```python
from build123d import *

# Parameters (mm, degrees)
F0_W     = 490
F0_H     = 6
F1_DEPTH = 50


# Not quite as in the source:
# - a feature names something its author has since deleted; it is built from what else it names
# - the program builds the solid bodies; features that only make, move or delete a surface that nothing else refers to are left out


with BuildPart() as f1:
    # F0 (on Top) → F1 (new body)
    with BuildSketch(Plane.XY):
        Polygon((0, 1190), (0, 0), (515, 0), (540, 0), (540, 25), (540, 125), (540, 131), (540, 539), (540, 545), (540, 645), (540, 651), (540, 1059), (540, 1065), (540, 1165), (540, 1190), (515, 1190), align=None)
        Polygon((25, 1065), (25, 1165), (515, 1165), (515, 1065), (515, 1059), (515, 651), (515, 645), (515, 545), (515, 539), (515, 131), (515, 125), (515, 25), (25, 25), (25, 125), (25, 131), (25, 539), (25, 545), (25, 645), (25, 651), (25, 1059), align=None, mode=Mode.SUBTRACT)
        Polygon((540, 25), (540, 0), (1030, 0), (1055, 0), (1055, 25), (1055, 125), (1055, 131), (1055, 539), (1055, 545), (1055, 645), (1055, 651), (1055, 1059), (1055, 1065), (1055, 1165), (1055, 1190), (1030, 1190), (540, 1190), (540, 1165), (1030, 1165), (1030, 1065), (1030, 1059), (1030, 651), (1030, 645), (1030, 545), (1030, 539), (1030, 131), (1030, 125), (1030, 25), align=None)
        Polygon((1055, 25), (1055, 0), (1545, 0), (1570, 0), (1570, 25), (1570, 125), (1570, 131), (1570, 539), (1570, 545), (1570, 645), (1570, 651), (1570, 1059), (1570, 1065), (1570, 1165), (1570, 1190), (1545, 1190), (1055, 1190), (1055, 1165), (1545, 1165), (1545, 1065), (1545, 1059), (1545, 651), (1545, 645), (1545, 545), (1545, 539), (1545, 131), (1545, 125), (1545, 25), align=None)
        Polygon((1570, 25), (1570, 0), (2085, 0), (2085, 1190), (1570, 1190), (1570, 1165), (2060, 1165), (2060, 1065), (2060, 1059), (2060, 651), (2060, 645), (2060, 545), (2060, 539), (2060, 131), (2060, 125), (2060, 25), align=None)
        with Locations((270, 542)):
            Rectangle(F0_W, F0_H)
        with Locations((270, 128)):
            Rectangle(F0_W, F0_H)
        with Locations((270, 648)):
            Rectangle(F0_W, F0_H)
        with Locations((270, 1062)):
            Rectangle(F0_W, F0_H)
        with Locations((785, 648)):
            Rectangle(F0_W, F0_H)
        with Locations((1300, 648)):
            Rectangle(F0_W, F0_H)
        with Locations((1300, 542)):
            Rectangle(F0_W, F0_H)
        with Locations((785, 542)):
            Rectangle(F0_W, F0_H)
        with Locations((1815, 542)):
            Rectangle(F0_W, F0_H)
        with Locations((1815, 648)):
            Rectangle(F0_W, F0_H)
        with Locations((1815, 1062)):
            Rectangle(F0_W, F0_H)
        with Locations((1300, 1062)):
            Rectangle(F0_W, F0_H)
        with Locations((785, 1062)):
            Rectangle(F0_W, F0_H)
        with Locations((1815, 128)):
            Rectangle(F0_W, F0_H)
        with Locations((785, 128)):
            Rectangle(F0_W, F0_H)
        with Locations((1300, 128)):
            Rectangle(F0_W, F0_H)
    extrude(amount=F1_DEPTH)


solid = f1.part
```
Geometry: final body of the model. Coordinates: model frame, mm. Coordinates: 2 decimals unless noted, no trailing zeros. Order: outer loops, then holes, each group sorted by start corner. A loop starts at its lowest first (then second) coordinate and runs counter-clockwise, first axis right, second up. Notation, with made-up numbers: (8.25, -25) - (64.25, -25) arc R20 cw to (64.25, 4) - close; hole circle Ø11 at (-4.5, 53). An arc over 180 degrees is marked (long way). Write each question's results on one line, items separated by ' | '.
1) Pull-direction query (X, two-part tool) for faces 1 (the flat face through (1038, 598, 50)), 2 (the flat face through (0, 603, 25)), 3 (the flat face through (267, 545, 25)); classes: pulls with the +X half, pulls with the -X half, needs draft (parallel to the pull), parting line crosses it, or undercut.
Results list:
face 1: needs draft | face 2: pulls with the -X half | face 3: undercut
2) Line query: line 1 (Y direction, x = 783, z = 3); line 2 (X direction, y = 1109, z = 24). Output: solid intervals per line, ascending. Write a range as from..to.
Results list:
line 1: 0..25, 125..131, 539..545, 645..651, 1059..1065, 1165..1190 | line 2: 0..25, 515..540, 1030..1055, 1545..1570, 2060..2085
3) Section A-A, the plane y = 238. Return loops of the section in (x, z).
Results list:
outline: (0, 0) - (25, 0) - (25, 50) - (0, 50) - close; (515, 0) - (540, 0) - (540, 50) - (515, 50) - close; (1030, 0) - (1055, 0) - (1055, 50) - (1030, 50) - close; (1545, 0) - (1570, 0) - (1570, 50) - (1545, 50) - close; (2060, 0) - (2085, 0) - (2085, 50) - (2060, 50) - close
4) Section B-B, the plane x = 561. Return loops of the section in (y, z), plus the area to 3 significant figures.
Results list:
outline: (0, 0) - (25, 0) - (25, 50) - (0, 50) - close; (125, 0) - (131, 0) - (131, 50) - (125, 50) - close; (539, 0) - (545, 0) - (545, 50) - (539, 50) - close; (645, 0) - (651, 0) - (651, 50) - (645, 50) - close; (1059, 0) - (1065, 0) - (1065, 50) - (1059, 50) - close; (1165, 0) - (1190, 0) - (1190, 50) - (1165, 50) - close | area: 3,700 mm^2
5) Section C-C, the plane z = 22. State how many separate pieces and enclosed holes the cut face has, plus the area to 3 significant figures.
Results list:
separate pieces: 1 | enclosed holes: 20 | area: 294,000 mm^2
